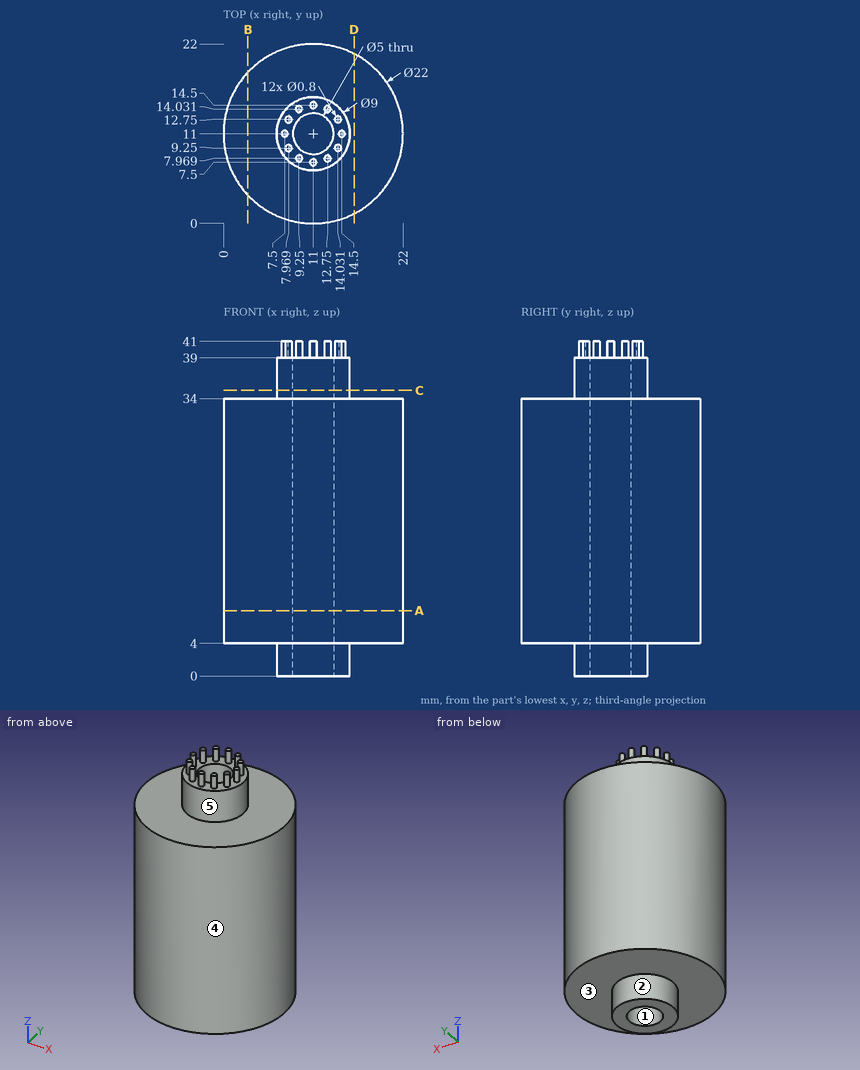
Print and shaded views of the part. All mm, measured from the part's lowest x, y and z. A direction names the side the tool comes from. Give positions to 0.01 mm unless a question says otherwise; leave off trailing zeros. Order: outer loops, then holes, each group sorted by start corner. A loop starts at its lowest first (then second) coordinate and runs counter-clockwise, first axis right, second up. Notation, with made-up numbers: M 24.25,-39.5 L 68.25,-39.5 A20 cw 68.25,-34.5 Z; hole C 50,7.5 d3. An arc over 180 degrees is marked long. Use one line per item in the form item = value.
Q1. Slice it at B-B, the plane x = 3. Write the cut outline in (y, z).
Conclusion:
outline = M 3.45,4 L 18.55,4 L 18.55,34 L 3.45,34 Z
Q2. Slice it at A-A, the plane z = 8. Write the cut outline in (x, y).
Conclusion:
outline = C 11,11 d22; hole C 11,11 d5
Q3. Pin check, flat tips, straight feed: P1, Ø3, axis at x = 18, y = 11, coming from the +Z side; P2, Ø2, axis at y = 17, z = 13, coming from the -X side; P3, Ø1.5, axis at x = 18.5, y = 15.5, coming from the -Z side. Stop position of each tip, or through.
Conclusion:
P1 = 34
P2 = 1.2
P3 = 4
Q4. Pull direction X, two halves, no side cores. Call the marked faces 1, 2 and 3: released by +X, released by -X, zero draft, split by the parting line, or undercut.
Conclusion:
face_1 = undercut
face_2 = split by the parting line
face_3 = zero draft
Q5. Slice it at C-C, the plane z = 35. Write the cut outline in (x, y).
Conclusion:
outline = C 11,11 d9; hole C 11,11 d5
Q6. Which spindle directions (+Z, -Z, +X, -X, +Y, -Y) get a long thin tool onto all of the face, cutting with end or side? Do the marked faces 4 and 5. Say none if no direction does.
Conclusion:
face_4 = +Z, -Z
face_5 = +Z
Q7. Wall check: probe 1 along Y at (x, z) = (11, 19); probe 2 along Z at (x, y) = (10, 5); probe 3 along Y at (x, z) = (9.25, 2.5) (1 decimal). Give the ranges that are in metal, low to high.
Conclusion:
probe_1 = 0 to 8.5, 13.5 to 22
probe_2 = 4 to 34
probe_3 = 6.9 to 9.2, 12.8 to 15.1
Q8. Slice it at D-D, the plane x = 16. Write the cut outline in (y, z), and give its area (3 significant figures).
Conclusion:
outline = M 1.2,4 L 20.8,4 L 20.8,34 L 1.2,34 Z
area = 588 mm2
